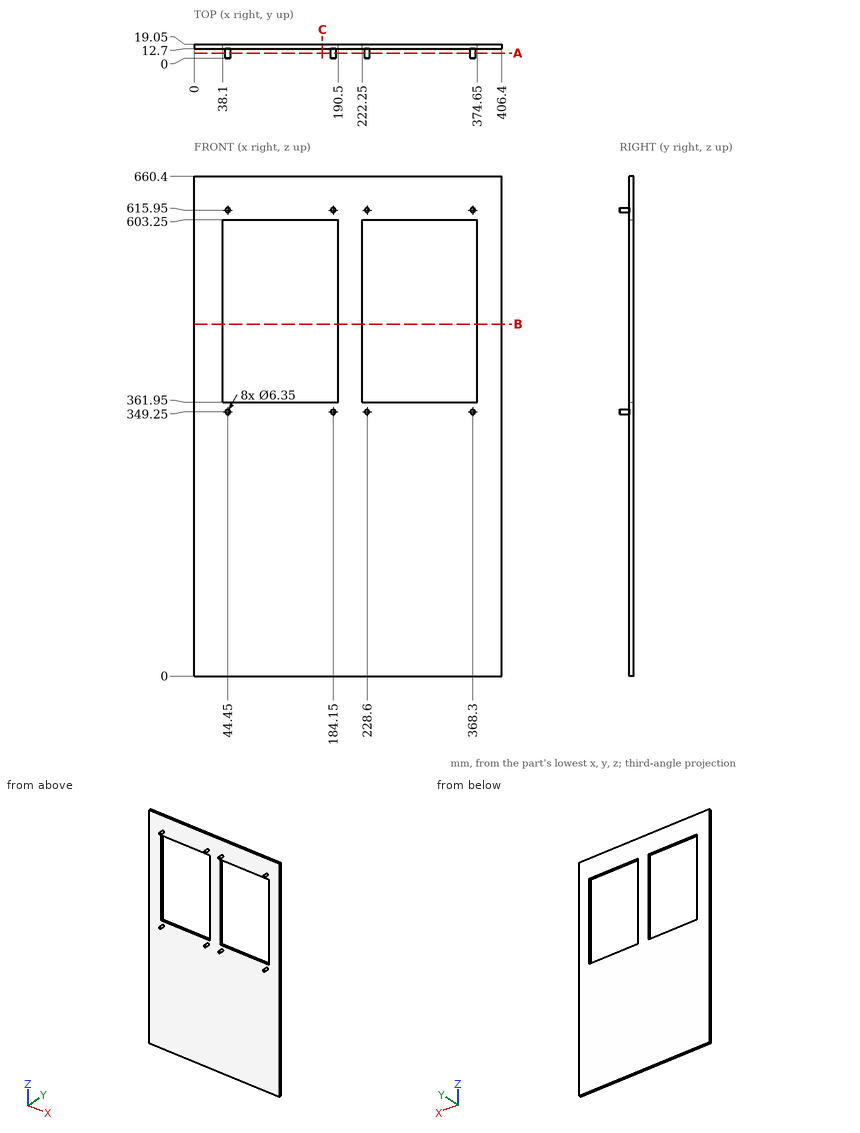
Verification items for this drawing (mm, ordinates from the low corner). Give positions to 0.01 mm unless a question says otherwise; leave off trailing zeros. Loops run counter-clockwise (first coordinate to the right, second up) from the corner with the lowest first, then second, coordinate; pieces in that order, holes last. Notation, with made-up numbers: M 14.5,0.25 L 64.5,0.25 A28 ccw 64.5,20.25 Z; hole C 70.5,-8 d6. An arc over 180 degrees is marked long. Write item = value, one per line. Start each with the question number.
1. Section check B-B, the plane z = 465. Enter the section's corners in (x, y), plus the area to 3 significant figures.
2. Section check C-C, the plane x = 169.5. Enter the section's corners in (y, z), plus the area to 3 significant figures.
3. Thickness scan on probe 1 along X at (y, z) = (13, 505); probe 2 along X at (y, z) = (11.25, 615); probe 3 along Z at (x, y) = (328.5, 17.5). Record the ranges inside material, lowest first.
4. Section check A-A, the plane y = 7. Enter the section's corners in (x, z) (3 decimals), plus the area to 3 significant figures.
Values follow:
q1.outline = M 0,12.7 L 38.1,12.7 L 38.1,19.05 L 0,19.05 Z; M 190.5,12.7 L 222.25,12.7 L 222.25,19.05 L 190.5,19.05 Z; M 374.65,12.7 L 406.4,12.7 L 406.4,19.05 L 374.65,19.05 Z
q1.area = 645 mm^2
q2.outline = M 12.7,0 L 19.05,0 L 19.05,361.95 L 12.7,361.95 Z; M 12.7,603.25 L 19.05,603.25 L 19.05,660.4 L 12.7,660.4 Z
q2.area = 2,660 mm^2
q3.probe_1 = 0 to 38.1, 190.5 to 222.25, 374.65 to 406.4
q3.probe_2 = 41.42 to 47.48, 181.12 to 187.18, 225.57 to 231.63, 365.27 to 371.33
q3.probe_3 = 0 to 361.95, 603.25 to 660.4
q4.outline = C 44.45,349.25 d6.35; C 44.45,615.95 d6.35; C 184.15,349.25 d6.35; C 184.15,615.95 d6.35; C 228.6,349.25 d6.35; C 228.6,615.95 d6.35; C 368.3,349.25 d6.35; C 368.3,615.95 d6.35
q4.area = 253 mm^2
